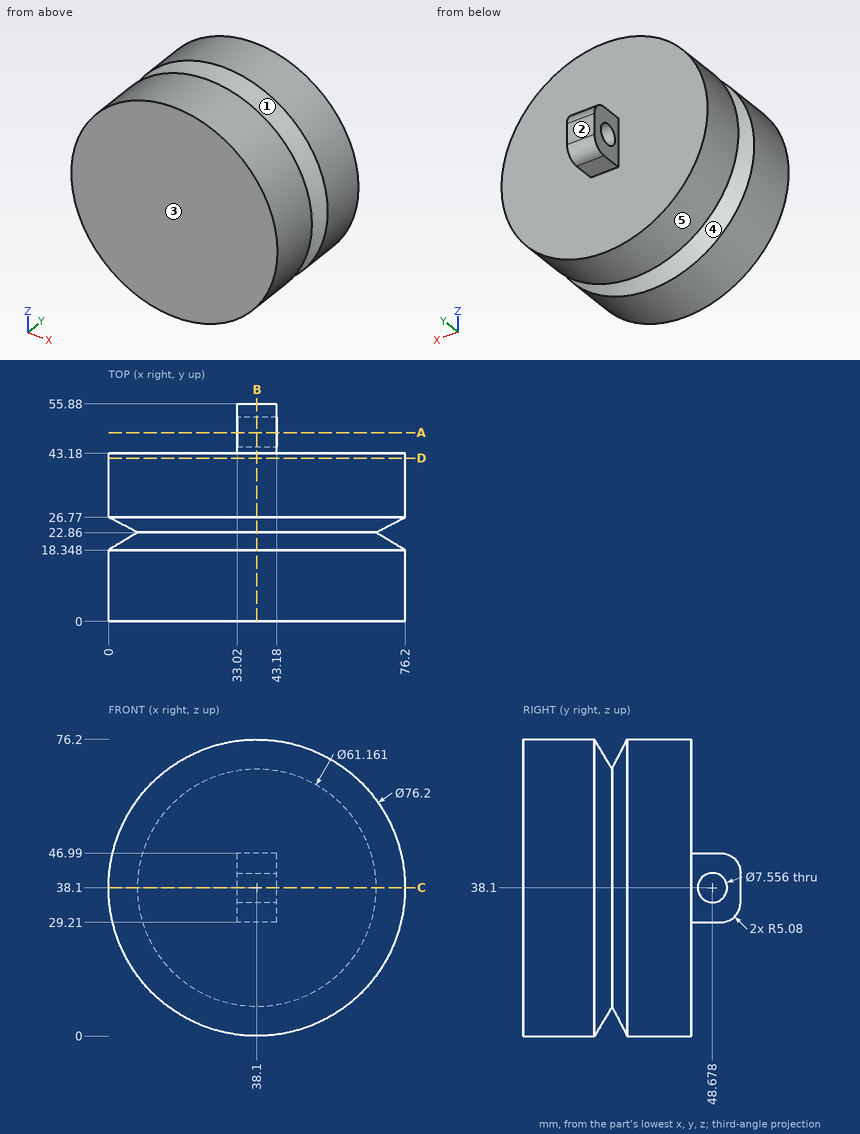
Check sheet for the drawn part. Datum: minimum x, y, z corner. Units: mm. A direction names the side the tool comes from. Coordinates: 2 decimals unless noted, no trailing zeros. Loops run counter-clockwise (first coordinate to the right, second up) from the corner with the lowest first, then second, coordinate; pieces in that order, holes last. Notation, with made-up numbers: (61.5, 35.5) -> (72.5, 35.5) arc R23 cw to (72.5, 71.5) -> close; hole circle Ø2 at (58.5, -32). An arc over 180 degrees is marked (long way). Answer as a JSON object with one key per item and string values. Group by question number.
Item 1: Mould release check, pull along Y, two halves, no side actions. Record for the marked faces 3, 4 and 5: +Y half, -Y half, draft (parallel to the pull), parting line (faces both ways), or undercut.
Item 2: Tool access check on the marked faces 1 and 2. Record the directions out of +Z, -Z, +X, -X, +Y, -Y that give a thin tool (end or side, any length) a straight path to the whole face; none if there is none.
Item 3: Scan lines: probe 1 along Z at (x, y) = (37.5, 42) (1 decimal); probe 2 along Y at (x, z) = (71.5, 31) (1 decimal); probe 3 along Y at (x, z) = (14, 19.5). Record each from-to range of solid material in increasing order.
Item 4: Sectioned sample at A-A on y = 48.5. Record the boundary of the cut face in (x, z).
Item 5: Sectioned sample at C-C on z = 38.1. Record the boundary of the cut face in (x, y), plus the area to 3 significant figures.
Item 6: Depth check by flat-ended pin: pin 1 (8 mm diameter, centred on y = 40.5, z = 48, fed in from +X); pin 2 (10 mm diameter, centred on y = 47.5, z = 37.5, fed in from +X); pin 3 (8 mm diameter, centred on y = 46.5, z = 51.5, fed in from +X) (1 decimal); pin 4 (5 mm diameter, centred on x = 60.5, y = 31.5, fed in from -Z). Enter the tip coordinate at first touch or a pass-through.
Item 7: Sectioned sample at D-D on y = 42. Record the boundary of the cut face in (x, z).
Item 8: Sectioned sample at B-B on x = 38.1. Record the boundary of the cut face in (y, z).
Evaluation:
{
 "1": {"face 3": "-Y half", "face 4": "undercut", "face 5": "draft"},
 "2": {"face 1": "none", "face 2": "+Z, -Z, +X, -X, +Y"},
 "3": {"probe 1": "z = 0 to 76.2", "probe 2": "y = 0 to 20.7, 24.7 to 43.2", "probe 3": "y = 0 to 43.18"},
 "4": {"outline": "(33.02, 29.21) -> (43.18, 29.21) -> (43.18, 34.33) -> (33.02, 34.33) -> close; (33.02, 41.87) -> (43.18, 41.87) -> (43.18, 46.99) -> (33.02, 46.99) -> close"},
 "5": {"outline": "(0, 0) -> (76.2, 0) -> (76.2, 18.35) -> (68.68, 22.86) -> (76.2, 26.77) -> (76.2, 43.18) -> (43.18, 43.18) -> (43.18, 44.9) -> (33.02, 44.9) -> (33.02, 43.18) -> (0, 43.18) -> (0, 26.77) -> (7.52, 22.86) -> (0, 18.35) -> close; (33.02, 52.46) -> (43.18, 52.46) -> (43.18, 55.88) -> (33.02, 55.88) -> close", "area": "3,280 mm²"},
 "6": {"pin 1": "stops at x = 75.74", "pin 2": "stops at x = 76.2", "pin 3": "stops at x = 74.5", "pin 4": "stops at z = 5.61"},
 "7": {"outline": "circle Ø76.2 at (38.1, 38.1)"},
 "8": {"outline": "(0, 0) -> (18.35, 0) -> (22.86, 7.52) -> (26.77, 0) -> (43.18, 0) -> (43.18, 29.21) -> (50.8, 29.21) arc R5.08 ccw to (55.88, 34.29) -> (55.88, 41.91) arc R5.08 ccw to (50.8, 46.99) -> (43.18, 46.99) -> (43.18, 76.2) -> (26.77, 76.2) -> (22.86, 68.68) -> (18.35, 76.2) -> (0, 76.2) -> close; hole circle Ø7.56 at (48.68, 38.1)"}
}
